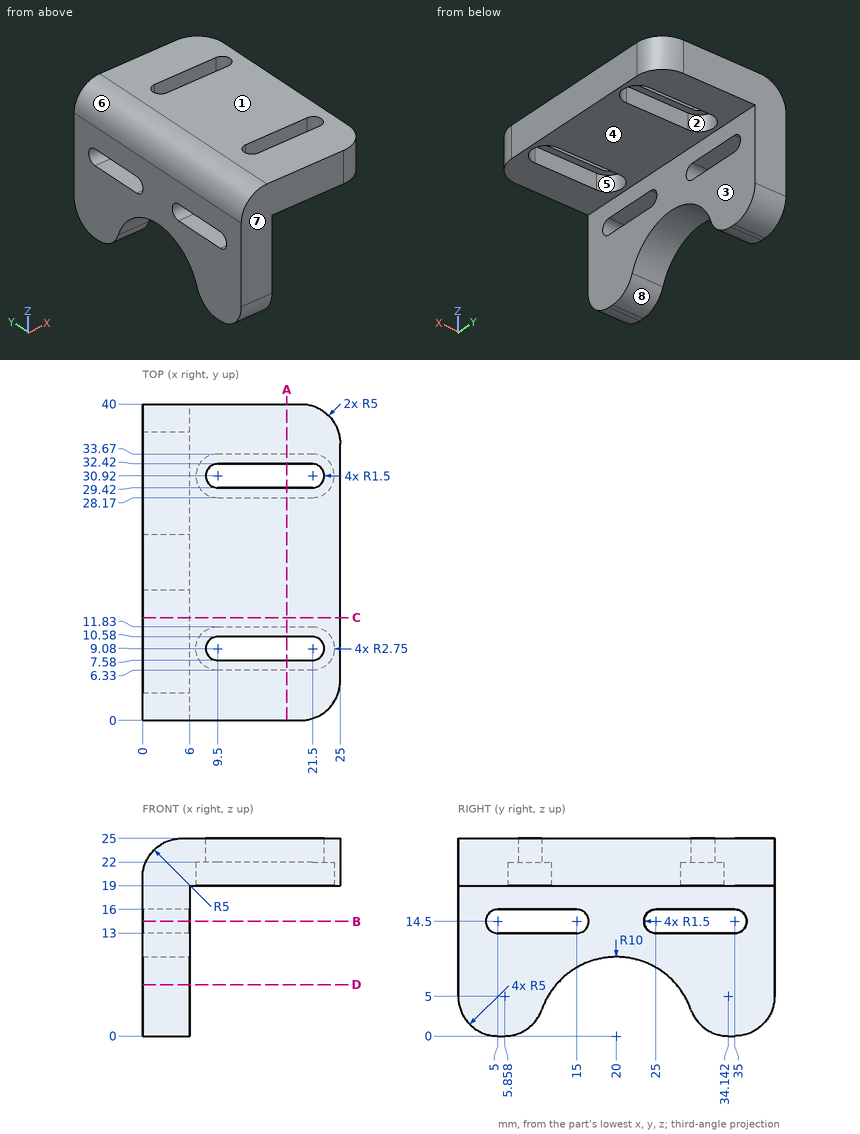
Input: dimensioned drawing with shaded views. Units: mm. Origin: part minimum x, y, z. A direction names the side the tool comes from. Give positions to 0.01 mm unless a question says otherwise; leave off trailing zeros. Write each loop counter-clockwise with the first axis right and the second up, starting at its lowest first coordinate (ties: lowest second). Pieces come first, ordered by that corner, then holes. Notation, with made-up numbers: (-32.75, 67) -> (-15.75, 67) arc R33 ccw to (-15.75, 106) -> close; hole circle Ø11 at (81, 82). An arc over 180 degrees is marked (long way). Return JSON: item names as keys, results as strings. Group by question number.
1. Pin query (flat end, axial travel): pin 1 Ø4 at (y, z) = (4.5, 9.5) entering from +X; pin 2 Ø5 at (x, y) = (2.5, 12.5) entering from -Z; pin 3 Ø4.5 at (x, y) = (16, 10) entering from -Z; pin 4 Ø3 at (y, z) = (17.5, 7) entering from +X. Return the tip coordinate at first contact, or that it passes through.
2. Section B-B, the plane z = 14.5. Output: boundary loops of the cut face in (x, y), then the cut area to 3 significant figures.
3. Section C-C, the plane y = 13. Output: boundary loops of the cut face in (x, z), then the cut area to 3 significant figures.
4. Section A-A, the plane x = 18.25. Output: boundary loops of the cut face in (y, z).
5. Material intervals for line 1 (Z direction, x = 18, y = 24); line 2 (X direction, y = 7.5, z = 5); line 3 (Y direction, x = 5.25, z = 15.5), sorted ascending. Write a range as from..to.
6. Access query for the marked faces 4, 5, 6, 7 and 8. Directions: +Z, -Z, +X, -X, +Y, -Y. A direction counts if a zero-diameter tool reaches every point of the face in a straight line with its end or side. Return the directions, or none.
7. Mould query, pull axis X, two halves, no side actions, for the marked faces 1, 2 and 3. Classes: +X half, -X half, draft (parallel to the pull), parting line (faces both ways), or undercut.
8. Section D-D, the plane z = 6.5. Output: boundary loops of the cut face in (x, y), then the cut area to 3 significant figures.
Determined:
{
 "1": {"pin 1": "stops at x = 6", "pin 2": "stops at z = 2.2", "pin 3": "stops at z = 19", "pin 4": "passes through"},
 "2": {"outline": "(0, 0) -> (6, 0) -> (6, 3.5) -> (0, 3.5) -> close; (0, 16.5) -> (6, 16.5) -> (6, 23.5) -> (0, 23.5) -> close; (0, 36.5) -> (6, 36.5) -> (6, 40) -> (0, 40) -> close", "area": "84.0 mm2"},
 "3": {"outline": "(0, 7.14) -> (6, 7.14) -> (6, 13) -> (0, 13) -> close; (0, 16) -> (6, 16) -> (6, 19) -> (25, 19) -> (25, 25) -> (5, 25) arc R5 ccw to (0, 20) -> close", "area": "198 mm2"},
 "4": {"outline": "(0, 19) -> (6.33, 19) -> (6.33, 22) -> (7.58, 22) -> (7.58, 25) -> (0, 25) -> close; (10.58, 22) -> (11.83, 22) -> (11.83, 19) -> (28.17, 19) -> (28.17, 22) -> (29.42, 22) -> (29.42, 25) -> (10.58, 25) -> close; (32.42, 22) -> (33.67, 22) -> (33.67, 19) -> (40, 19) -> (40, 25) -> (32.42, 25) -> close"},
 "5": {"line 1": "z = 19..25", "line 2": "x = 0..6", "line 3": "y = 0..3.88, 16.12..23.88, 36.12..40"},
 "6": {"face 4": "-Z, +X, +Y, -Y", "face 5": "-Z", "face 6": "+Z, -X, +Y, -Y", "face 7": "+Z, -Z, +X, -X, -Y", "face 8": "-Z, +X, -X"},
 "7": {"face 1": "draft", "face 2": "undercut", "face 3": "+X half"},
 "8": {"outline": "(0, 0) -> (6, 0) -> (6, 12.4) -> (0, 12.4) -> close; (0, 27.6) -> (6, 27.6) -> (6, 40) -> (0, 40) -> close", "area": "149 mm2"}
}
